Geometry: final body of the model. Coordinates: model frame, mm. A direction names the side the tool comes from. Round coordinates to 2 decimals unless told otherwise and drop trailing zeros. Order: outer loops, then holes, each group sorted by start corner. A loop starts at its lowest first (then second) coordinate and runs counter-clockwise, first axis right, second up. Notation, with made-up numbers: (53.25, 9.5) - (70.25, 9.5) arc R21 ccw to (70.25, 34.5) - close; hole circle Ø5 at (74.25, 58). An arc over 180 degrees is marked (long way). Put each result on its own line as item: value. Start each with the question number.
(1) Pin query (flat end, axial travel): P1, Ø1.2, axis at x = 190.5, y = 38.5, coming from the -Z side; P2, Ø3, axis at x = 132.5, y = 87, coming from the -Z side; P3, Ø1, axis at y = 68.5, z = 1.5, coming from the +X side; P4, Ø2, axis at x = 192.6, y = 18.64, coming from the +Z side. Return the tip coordinate at first contact, or that it passes through.
(2) Material intervals for L1, parallel to X at y = 38, z = 5.5; L2, parallel to X at y = 37, z = 4; L3, parallel to Z at x = 189.5, y = 81, sorted ascending. Write a range as [from, to].
(3) Section B-B (x = 168). Output: boundary loops of the cut face in (y, z).
(4) Pull-direction query (X, two-part tool) for faces 1 (the face through (156, 92.137, 5)), 2 (the face through (196.6, 53, 5)), 3 (the face through (116.5, 42.74, 0.86)), 4 (the face through (195.46, 19.54, 4.82)); classes: released by +X, released by -X, zero draft, split by the parting line, or undercut.
(5) Section C-C (y = 81.5). Output: boundary loops of the cut face in (x, z), and give its area (3 significant figures).
(6) Section A-A (z = 2). Output: boundary loops of the cut face in (x, y).
(7) Access query for faces 5 (the face through (193.984, 64.975, 4.821)), 6 (the face through (156, 82, 3.3)), 7 (the face through (130, 87, 4.8)), 8 (the face through (191.68, 19.48, 1.63)), 9 (the face through (156, 14.637, 5)). Directions: +Z, -Z, +X, -X, +Y, -Y. A direction counts if a zero-diameter tool reaches every point of the face in a straight line with its end or side. Return the directions, or none.
from build123d import *

# Parameters (mm, degrees)
SKETCH1_W           = 81
SKETCH1_H           = 57
SKETCH1_R           = 1.25
BOSS_EXTRUDE1_DEPTH = 3.3
SKETCH2_W           = 81
SKETCH2_H           = 77.5
SKETCH2_R           = 1.25
BOSS_EXTRUDE2_DEPTH = 3
CUT_EXTRUDE1_DEPTH  = 218.210667029
SKETCH4_R           = 6
CUT_EXTRUDE2_DEPTH  = 3.3
CUT_EXTRUDE3_DEPTH  = 1.5
SKETCH6_R           = 3
CUT_EXTRUDE4_DEPTH  = 3
FILLET1_R           = 3


with BuildPart() as part:
    # Sketch1 → Boss-Extrude1 (new body)
    with BuildSketch(Plane.XY):
        with Locations((156.100114143, 43.136740717)):
            Rectangle(SKETCH1_W, SKETCH1_H)
        with Locations((192.600114143, 18.636740717)):
            Circle(SKETCH1_R, mode=Mode.SUBTRACT)
        with Locations((192.600114143, 67.636740717)):
            Circle(SKETCH1_R, mode=Mode.SUBTRACT)
    extrude(amount=BOSS_EXTRUDE1_DEPTH)

    # Sketch2 → Boss-Extrude2 (add)
    with BuildSketch(Plane.XY.offset(3.3)):
        with Locations((156.100114143, 53.386740717)):
            Rectangle(SKETCH2_W, SKETCH2_H)
        with Locations((192.600114143, 67.636740717)):
            Circle(SKETCH2_R, mode=Mode.SUBTRACT)
        with Locations((192.600114143, 18.636740717)):
            Circle(SKETCH2_R, mode=Mode.SUBTRACT)
    extrude(amount=BOSS_EXTRUDE2_DEPTH)

    # Sketch3 → Cut-Extrude1 (cut, through all)
    with BuildSketch(Plane.XY.offset(6.3)):
        with BuildLine():
            Line((131.600114143, 85.886740717), (131.600114143, 87.136740717))
            Line((131.600114143, 87.136740717), (132.850114143, 87.136740717))
            ThreePointArc((132.850114143, 87.136740717), (130.716230667, 88.020624193), (131.600114143, 85.886740717))
        make_face()
        with BuildLine():
            Line((132.850114143, 87.136740717), (131.600114143, 87.136740717))
            Line((131.600114143, 87.136740717), (131.600114143, 85.886740717))
            ThreePointArc((131.600114143, 85.886740717), (132.48399762, 86.25285724), (132.850114143, 87.136740717))
        make_face()
        with BuildLine():
            ThreePointArc((190.850114143, 87.136740717), (189.600114143, 88.386740717), (188.350114143, 87.136740717))
            Line((188.350114143, 87.136740717), (189.600114143, 87.136740717))
            Line((189.600114143, 87.136740717), (189.600114143, 85.886740717))
            ThreePointArc((189.600114143, 85.886740717), (190.48399762, 86.25285724), (190.850114143, 87.136740717))
        make_face()
        with BuildLine():
            Line((189.600114143, 87.136740717), (188.350114143, 87.136740717))
            ThreePointArc((188.350114143, 87.136740717), (188.716230667, 86.25285724), (189.600114143, 85.886740717))
            Line((189.600114143, 85.886740717), (189.600114143, 87.136740717))
        make_face()
        with BuildLine():
            ThreePointArc((190.850114143, 38.136740717), (190.48399762, 39.020624193), (189.600114143, 39.386740717))
            Line((189.600114143, 39.386740717), (189.600114143, 38.136740717))
            Line((189.600114143, 38.136740717), (188.350114143, 38.136740717))
            ThreePointArc((188.350114143, 38.136740717), (189.600114143, 36.886740717), (190.850114143, 38.136740717))
        make_face()
        with BuildLine():
            Line((189.600114143, 38.136740717), (189.600114143, 39.386740717))
            ThreePointArc((189.600114143, 39.386740717), (188.716230667, 39.020624193), (188.350114143, 38.136740717))
            Line((188.350114143, 38.136740717), (189.600114143, 38.136740717))
        make_face()
        with BuildLine():
            ThreePointArc((132.850114143, 38.136740717), (132.48399762, 39.020624193), (131.600114143, 39.386740717))
            Line((131.600114143, 39.386740717), (131.600114143, 38.136740717))
            Line((131.600114143, 38.136740717), (132.850114143, 38.136740717))
        make_face()
        with BuildLine():
            Line((131.600114143, 38.136740717), (131.600114143, 39.386740717))
            ThreePointArc((131.600114143, 39.386740717), (130.716230667, 37.25285724), (132.850114143, 38.136740717))
            Line((132.850114143, 38.136740717), (131.600114143, 38.136740717))
        make_face()
    extrude(amount=-CUT_EXTRUDE1_DEPTH, mode=Mode.SUBTRACT)

    # Sketch4 → Cut-Extrude2 (cut)
    with BuildSketch(Plane(origin=(0, 0, 0), x_dir=(-1, 0, 0), z_dir=(0, 0, -1))):
        with Locations((-189.600114143, 38.136740717)):
            Circle(SKETCH4_R)
        with Locations((-131.600114143, 38.136740717)):
            Circle(SKETCH4_R)
    extrude(amount=-CUT_EXTRUDE2_DEPTH, mode=Mode.SUBTRACT)

    # Sketch5 → Cut-Extrude3 (cut)
    with BuildSketch(Plane(origin=(0, 0, 3.3), x_dir=(-1, 0, 0), z_dir=(0, 0, -1))):
        Polygon((-187.290713067, 87.136740717), (-188.445413605, 89.136740717), (-190.754814682, 89.136740717), (-191.90951522, 87.136740717), (-190.754814682, 85.136740717), (-188.445413605, 85.136740717), align=None)
        Polygon((-129.290713067, 87.136740717), (-130.445413605, 89.136740717), (-132.754814682, 89.136740717), (-133.90951522, 87.136740717), (-132.754814682, 85.136740717), (-130.445413605, 85.136740717), align=None)
        Polygon((-130.445413605, 40.136740717), (-132.754814682, 40.136740717), (-133.90951522, 38.136740717), (-132.754814682, 36.136740717), (-130.445413605, 36.136740717), (-129.290713067, 38.136740717), align=None)
        Polygon((-187.290713067, 38.136740717), (-188.445413605, 40.136740717), (-190.754814682, 40.136740717), (-191.90951522, 38.136740717), (-190.754814682, 36.136740717), (-188.445413605, 36.136740717), align=None)
    extrude(amount=-CUT_EXTRUDE3_DEPTH, mode=Mode.SUBTRACT)

    # Sketch6 → Cut-Extrude4 (cut)
    with BuildSketch(Plane.XY.offset(6.3)):
        with Locations((192.600114143, 67.636740717)):
            Circle(SKETCH6_R)
        with Locations((192.600114143, 18.636740717)):
            Circle(SKETCH6_R)
    extrude(amount=-CUT_EXTRUDE4_DEPTH, mode=Mode.SUBTRACT)

    # Fillet1
    # the kernel refuses this fillet: 3 mm, written as the material it takes off along each edge
    with BuildSketch(Plane(origin=(108.100114143, 71.636740717, 0), x_dir=(0, 0, 1), z_dir=(1, 0, 0))) as fillet1_piece_1:
        with BuildLine():
            CenterArc((FILLET1_R, FILLET1_R), FILLET1_R, 180, 90)
            Line((0, FILLET1_R), (0, 0))
            Line((0, 0), (FILLET1_R, 0))
        make_face()
    extrude(amount=96, mode=Mode.SUBTRACT)
    with BuildSketch(Plane(origin=(196.600114143, 79.136740717, 0), x_dir=(0, 0, 1), z_dir=(0, -1, 0)), Plane(origin=(115.600114143, 7.136740717, 0), x_dir=(0, 0, 1), z_dir=(0, 1, 0))) as fillet1_piece_2:
        with BuildLine():
            CenterArc((FILLET1_R, FILLET1_R), FILLET1_R, 180, 90)
            Line((0, FILLET1_R), (0, 0))
            Line((0, 0), (FILLET1_R, 0))
        make_face()
    extrude(amount=72, mode=Mode.SUBTRACT)
    with BuildSketch(Plane(origin=(204.100114143, 14.636740717, 0), x_dir=(0, 1, 0), z_dir=(-1, 0, 0))) as fillet1_piece_3:
        with BuildLine():
            CenterArc((FILLET1_R, -FILLET1_R), FILLET1_R, 90, 90)
            Line((0, -FILLET1_R), (0, 0))
            Line((0, 0), (FILLET1_R, 0))
        make_face()
    extrude(amount=96, mode=Mode.SUBTRACT)


solid = part.part
Checks:
1. P1: stops at z = 4.8
1. P2: stops at z = 3.3
1. P3: stops at x = 196.43
1. P4: passes through
2. L1: x = [115.6, 130.36], [132.84, 188.36], [190.84, 196.6]
2. L2: x = [115.6, 129.95], [133.25, 187.95], [191.25, 196.6]
2. L3: z = [3.3, 6.3]
3. outline: (14.64, 3) arc R3 ccw to (17.64, 0) - (68.64, 0) arc R3 ccw to (71.64, 3) - (71.64, 3.3) - (92.14, 3.3) - (92.14, 6.3) - (14.64, 6.3) - close
4. face 1: zero draft
4. face 2: released by +X
4. face 3: released by -X
4. face 4: undercut
5. outline: (115.6, 3.3) - (196.6, 3.3) - (196.6, 6.3) - (115.6, 6.3) - close
5. area: 243 mm²
6. outline: (115.77, 14.81) - (196.43, 14.81) - (196.43, 71.47) - (115.77, 71.47) - close; hole circle Ø12 at (131.6, 38.14); hole circle Ø12 at (189.6, 38.14); hole circle Ø2.5 at (192.6, 18.64); hole circle Ø2.5 at (192.6, 67.64)
7. face 5: +Z
7. face 6: -Z, +X, -X, +Y
7. face 7: -Z
7. face 8: +Z, -Z
7. face 9: +Z, -Z, +X, -X, -Y
